Autodesk Inventor part; units mm, degrees
ref_plane "YZ Plane" through (0, 0, 0) normal (1, 0, 0) x (0, 1, 0)
ref_plane "XZ Plane" through (0, 0, 0) normal (0, 1, 0) x (-1, 0, 0)
ref_plane "XY Plane" through (0, 0, 0) normal (0, 0, 1) x (1, 0, 0)
sketch "Sketch1" plane through (0, 0, 0) normal (0, 0, 1) x (1, 0, 0)
  line L0 (-25, 25) -> (25, 25)
  line L1 (25, 25) -> (25, -25)
  line L2 (25, -25) -> (-25, -25)
  line L3 (-25, -25) -> (-25, 25)
  circle A0 centre (-25, 25) radius 1.25
  circle A1 centre (-25, 25) radius 3
  circle A2 centre (-25, -25) radius 3
  circle A3 centre (-25, -25) radius 1.25
  circle A4 centre (25, -25) radius 3
  circle A5 centre (25, -25) radius 1.25
  circle A6 centre (25, 25) radius 3
  circle A7 centre (25, 25) radius 1.25
  circle A8 centre (0, 0) radius 45
  line L4 (27.8, 27.8) -> (-27.8, 27.8)
  line L5 (-27.8, 27.8) -> (-27.8, -27.8)
  line L6 (-27.8, -27.8) -> (27.8, -27.8)
  line L7 (27.8, -27.8) -> (27.8, 27.8)
  point P0 (-22, 25)
  point P1 (22, 25)
  point P2 (25, 22)
  point P3 (25, -22)
  point P4 (22, -25)
  point P5 (-22, -25)
  point P6 (-25, -22)
  point P7 (-25, 22)
  point P8 (-23.923, 27.8)
  point P9 (23.923, 27.8)
  point P10 (27.8, 23.923)
  point P11 (27.8, -23.923)
  point P12 (23.923, -27.8)
  point P13 (-23.923, -27.8)
  point P14 (-27.8, -23.923)
  point P15 (-27.8, 23.923)
  dimension "d0" = 50
  dimension "d1" = 25
  dimension "d2" = 50
  dimension "d3" = 25
  dimension "d4" = 2.5
  dimension "d5" = 6
  dimension "d8" = 360
  dimension "d12" = 90
  dimension "d14" = 2.8
extrude "Extrusion1" add sketch "Sketch1" along normal blind 3.5 contours A0 L3 A1 L5 L4 L0 | L0 A1 L3 A0 | A6 L4 L7 L1 A7 L0 | L0 A7 L1 A6 | L4 A1 | A2 L2 A3 L3 | L3 A3 L2 A2 L6 L5 | A1 L5 | A6 L4 | A1 L5 L4 | L5 A2 | L4 L7 A6 | A4 L7 L6 L2 A5 L1 | L1 A5 L2 A4 | L7 A6 | A2 L6 | A2 L6 L5 | A4 L7 | L6 A4 | L7 L6 A4 | A8
chamfer "Chamfer1" distance 2 angle 45 8 edges at (-23.923, -27.8, 1.75) (-27.8, -23.923, 1.75) (23.923, -27.8, 1.75) (27.8, -23.923, 1.75) (23.923, 27.8, 1.75) (27.8, 23.923, 1.75) (-23.923, 27.8, 1.75) (-27.8, 23.923, 1.75)
sketch "Sketch2" plane through (0, 0, 3.5) normal (0, 0, 1) x (1, 0, 0)
  circle A0 centre (0, 0) radius 37.25
  dimension "d18" = 74.5
extrude "Extrusion2" cut sketch "Sketch2" against normal blind 1.6
sketch "Sketch3" plane through (0, 0, 0) normal (0, 0, -1) x (-1, 0, 0)
  circle A0 centre (-17.9346, -27.7011) radius 1.65
  circle A1 centre (15.0226, -29.3824) radius 1.65
  circle A2 centre (15.0226, -29.3824) radius 1.65
  circle A3 centre (32.9571, -1.6813) radius 1.65
  circle A4 centre (17.9346, 27.7011) radius 1.65
  circle A5 centre (-15.0226, 29.3824) radius 1.65
  circle A6 centre (-32.9571, 1.6813) radius 1.65
  circle A7 centre (-17.9346, -27.7011) radius 1.65
  point P0 (0, 0)
  dimension "d23" = 360
equation "\"d2\" = d0"
properties part number "moteus_x1_mount"
The listing builds one solid part. Answer for the finished solid, in the listing's coordinates (mm). A direction names the side the tool comes from. Round coordinates to 2 decimals unless told otherwise and drop trailing zeros. Loops run counter-clockwise (first coordinate to the right, second up) from the corner with the lowest first, then second, coordinate; pieces in that order, holes last.
Q1. Find the intervals of material crossed by line 1 (Y direction, x = 0, z = 2.4); line 2 (Y direction, x = 25, z = 1.05), in increasing order.
Q2. Section C-C, the plane y = -25 is taken. Determine the outline of the cut face in (x, z), then the cut area to 3 significant figures.
Q3. For a pull along X with two mould halves and no side action, classify faces 1 (the face through (-1, -29, 0)), 2 (the face through (20.765, 39.923, 1.726)), 3 (the face through (22.92, 22.84, 0.94)) as released by +X, released by -X, zero draft, split by the parting line, or undercut.
Q4. Section A-A, the plane x = 0 is taken. Determine the outline of the cut face in (y, z), then the cut area to 3 significant figures.
Q5. Given pin 1 Ø4 at (x, y) = (-25, 25) entering from +Z; pin 2 Ø3 at (x, y) = (25, -25) entering from +Z; pin 3 Ø2 at (x, z) = (7.5, 2.5) entering from -Y; pin 4 Ø1.5 at (y, z) = (2.5, 1) entering from -X, each flat-ended and moving along its own axis, determine where each tip first touches the part or whether it passes through.
Q6. Which of the six approach directions +Z, -Z, +X, -X, +Y, -Y give full straight-line access (tool end or side, diameter ignored) to faces 4 (the face through (26.155, 25.479, 0.937)), 5 (the face through (0, 31, 1.9))?
Completed:
1. line 1: y = -45 to -37.25, 37.25 to 45
1. line 2: y = -37.42 to -26.25, -23.75 to -22, 22 to 23.75, 26.25 to 37.42
2. outline: (-37.42, 0) - (-26.25, 0) - (-26.25, 1.9) - (-27.61, 1.9) - (-27.61, 3.5) - (-37.42, 3.5) - close; (-23.75, 0) - (-22, 0) - (-22, 1.9) - (-23.75, 1.9) - close; (22, 0) - (23.75, 0) - (23.75, 1.9) - (22, 1.9) - close; (26.25, 0) - (37.42, 0) - (37.42, 3.5) - (27.61, 3.5) - (27.61, 1.9) - (26.25, 1.9) - close
2. area: 80.4 mm2
3. face 1: zero draft
3. face 2: split by the parting line
3. face 3: undercut
4. outline: (-45, 0) - (-27.8, 0) - (-27.8, 1.9) - (-37.25, 1.9) - (-37.25, 3.5) - (-45, 3.5) - close; (27.8, 0) - (45, 0) - (45, 3.5) - (37.25, 3.5) - (37.25, 1.9) - (27.8, 1.9) - close
4. area: 90.2 mm2
5. pin 1: stops at z = 3.5
5. pin 2: stops at z = 1.9
5. pin 3: stops at y = -44.53
5. pin 4: stops at x = -44.97
6. face 4: +Z, -Z
6. face 5: +Z
